Check sheet for the modelled part. Datum: model origin and axes. Units: mm. A direction names the side the tool comes from. Coordinates: 2 decimals unless noted, no trailing zeros. Loops run counter-clockwise (first coordinate to the right, second up) from the corner with the lowest first, then second, coordinate; pieces in that order, holes last. Notation, with made-up numbers: (-4, 31.25) - (2, 31.25) arc R19 ccw to (2, 53.25) - close; hole circle Ø8 at (49.25, 27). An arc over 180 degrees is marked (long way). Use a Markdown table: item, result. Add a question column.
1) Sectioned sample at A-A, the plane x = 0. Enter the section's corners in (y, z) (1 decimal), then the cut area to 3 significant figures.
2) Tool access check on faces 4 (the cylindrical face through (-0.853, 3.843, 3.914)), 5 (the flat face through (-2, 2, 0)). Record the directions out of +Z, -Z, +X, -X, +Y, -Y that give a thin tool (end or side, any length) a straight path to the whole face; none if there is none.
3) Sectioned sample at C-C, the plane z = 5.75. Enter the section's corners in (x, y).
4) Draft check along Y on faces 1 (the cylindrical face through (2.326, 0.732, 3.541)), 2 (the cylindrical face through (-3.78, 2.9, 0.39)), 3 (the flat face through (2.2, 1.5, 6.985)). Enter one of: pulls with the +Y half, pulls with the -Y half, needs draft (parallel to the pull), parting line crosses it, or undercut.
5) Thickness scan on line 1 (Y direction, x = 0, z = 1.75); line 2 (Y direction, x = 2, z = 5.5); line 3 (X direction, y = -1, z = 1.25). Record the ranges inside material, lowest first.
6) Sectioned sample at D-D, the plane z = 0.5. Enter the section's corners in (x, y) (1 decimal), then the cut area to 3 significant figures.
7) Go/stop test with flat-tipped pins: P1, Ø1, axis at x = 3, z = 3.5, coming from the -Y side; P2, Ø2, axis at x = -2, z = 6, coming from the +Y side; P3, Ø2, axis at x = 0, y = 0.5, coming from the +Z side; P4, Ø3, axis at x = -3, y = -3.5, coming from the -Z side. Record where each tip stops, or that it passes through.
from build123d import *

# Parameters (mm, degrees)
F2_R     = 2.4384
F3_DEPTH = 6.985


with BuildPart() as f1:
    # F0 (on Front) → F1 (revolve)
    with BuildSketch(Plane.XZ):
        with BuildLine():
            Line((0, 6.985), (0, 0))
            Line((0, 0), (4.7625, 0))
            Line((4.7625, 0), (4.7625, 0.77))
            Line((4.7625, 0.77), (3.937, 1.27))
            Line((3.937, 1.27), (3.937, 6.485))
            ThreePointArc((3.937, 6.485), (3.790553, 6.838553), (3.437, 6.985))
            Line((3.437, 6.985), (0, 6.985))
        make_face()
    revolve(axis=Axis((0, 0, 3.4925), (0, 0, -1)))

    # F2 (on face) → F3 (cut, through all)
    with BuildSketch(Plane.XY.offset(6.985)):
        Circle(F2_R)
    extrude(amount=-F3_DEPTH, mode=Mode.SUBTRACT)


solid = f1.part
Solved:
| question | item | result |
|---|---|---|
| 1 | outline | (-4.8, 0) - (-2.4, 0) - (-2.4, 7) - (-3.4, 7) arc R0.5 ccw to (-3.9, 6.5) - (-3.9, 1.3) - (-4.8, 0.8) - close; (2.4, 0) - (4.8, 0) - (4.8, 0.8) - (3.9, 1.3) - (3.9, 6.5) arc R0.5 ccw to (3.4, 7) - (2.4, 7) - close |
| 1 | area | 22.5 mm2 |
| 2 | face 4 | +Z |
| 2 | face 5 | -Z, +X, -X, +Y, -Y |
| 3 | outline | circle Ø7.87 at (0, 0); hole circle Ø4.88 at (0, 0) |
| 4 | face 1 | undercut |
| 4 | face 2 | parting line crosses it |
| 4 | face 3 | needs draft |
| 5 | line 1 | y = -3.94 to -2.44, 2.44 to 3.94 |
| 5 | line 2 | y = -3.39 to -1.39, 1.39 to 3.39 |
| 5 | line 3 | x = -3.84 to -2.22, 2.22 to 3.84 |
| 6 | outline | circle Ø9.5 at (0, 0); hole circle Ø4.9 at (0, 0) |
| 6 | area | 52.6 mm2 |
| 7 | P1 | stops at y = -3.04 |
| 7 | P2 | stops at y = 3.81 |
| 7 | P3 | passes through |
| 7 | P4 | stops at z = 0 |
